Autodesk Inventor part; units mm, degrees
ref_plane "Work Plane1" through (0, 19.05, 0) normal (0, 1, 0) x (-1, 0, 0)
ref_plane "YZ Plane" through (0, 0, 0) normal (1, 0, 0) x (0, 1, 0)
ref_plane "XY Plane" through (0, 0, 0) normal (0, 0, 1) x (1, 0, 0)
sketch "Sketch1" plane through (0, 0, 0) normal (0, 0, 1) x (1, 0, 0)
  line L0 (-106.628, 0) -> (106.628, 0) construction
  line L1 (-63.5, 19.05) -> (63.5, 19.05)
  line L2 (63.5, 19.05) -> (63.5, 15.875)
  line L3 (-63.5, 15.875) -> (-63.5, 19.05)
  line L4 (-63.5, 15.875) -> (-53.34, 15.875)
  line L5 (-53.34, 15.875) -> (-53.34, 16.891)
  line L6 (-53.34, 16.891) -> (-50.8, 16.891)
  line L7 (-50.8, 16.891) -> (-50.8, 15.875)
  line L8 (-50.8, 15.875) -> (0, 15.875)
  line L9 (0, 0) -> (0, 19.05) construction
  line L10 (63.5, 15.875) -> (53.34, 15.875)
  line L11 (53.34, 15.875) -> (53.34, 16.891)
  line L12 (53.34, 16.891) -> (50.8, 16.891)
  line L13 (50.8, 16.891) -> (50.8, 15.875)
  line L14 (50.8, 15.875) -> (0, 15.875)
  dimension "d0" = 127
  dimension "d1" = 38.1
  dimension "d2" = 31.75
  dimension "d3" = 10.16
  dimension "d4" = 2.54
  dimension "d5" = 1.016
revolve "Revolution1" add sketch "Sketch1" angle 360 about axis through (-106.628, 0, 0) along (1, 0, 0)
ref_plane "Work Plane1" through (0, 19.05, 0) normal (0, 1, 0) x (-1, 0, 0)
sketch "Sketch2" plane through (0, 19.05, 0) normal (0, 1, 0) x (-1, 0, 0)
  line L0 (-31.75, 0) -> (9.525, 0) construction
  line L1 (-31.75, -4.7625) -> (9.525, -4.7625)
  line L2 (9.525, 4.7625) -> (-31.75, 4.7625)
  arc A0 (-31.75, 4.7625) -> (-31.75, -4.7625) centre (-31.75, 0) ccw
  arc A1 (9.525, -4.7625) -> (9.525, 4.7625) centre (9.525, 0) ccw
  line L3 (-63.5, 19.05) -> (-63.5, -19.05)
  line L4 (-27.6225, 1.5875) -> (-27.6225, -1.5875)
  line L5 (5.3975, 1.5875) -> (5.3975, -1.5875)
  arc A2 (5.3975, 1.5875) -> (2.2225, 4.7625) centre (2.2225, 1.5875) ccw
  arc A3 (2.2225, -4.7625) -> (5.3975, -1.5875) centre (2.2225, -1.5875) ccw
  arc A4 (-24.4475, 4.7625) -> (-27.6225, 1.5875) centre (-24.4475, 1.5875) ccw
  arc A5 (-27.6225, -1.5875) -> (-24.4475, -4.7625) centre (-24.4475, -1.5875) ccw
  point P0 (0, 0)
  point P1 (-11.1125, 0)
  point P2 (-36.5125, 0)
  point P3 (9.525, 0)
  point P4 (-63.5, 0)
  dimension "d7" = 9.525
  dimension "d8" = 41.275
  dimension "d10" = 33.02
  dimension "d11" = 16.51
  dimension "d12" = 3.175
  dimension "d13" = 3.175
  dimension "d27" = 31.75
extrude "Extrusion1" cut sketch "Sketch2" against normal blind 2.032
extrude "Extrusion2" cut sketch "Sketch2" against normal up to surface contours A5 L4 A4 L2 A2 L5 A3 L1
hole "Hole1" at (-9.525, 19.05, 0) at (31.75, 19.05, 0) direction (0, -1, 0) diameter 2.1565 depth 6.35 tip angle 118
thread "Thread1"
properties part number "InventorNativeNewHilt" material "Aluminum 6061"
CAD build for the part. Positions are in the model's coordinates, mm. A direction names the side the tool comes from. Coordinates: 2 decimals unless noted, no trailing zeros. Loops run counter-clockwise (first coordinate to the right, second up) from the corner with the lowest first, then second, coordinate; pieces in that order, holes last. Notation, with made-up numbers: (-32.5, 22.25) - (-15.5, 22.25) arc R8 cw to (-15.5, 35.25) - close; hole circle Ø5 at (60, 18.5). An arc over 180 degrees is marked (long way). Return JSON: item names as keys, results as strings.
1. Drop flat-ended pins along their axis: pin 1 (1.7 mm diameter, centred on x = 10.5, y = 17, fed in from -Z); pin 2 (6 mm diameter, centred on x = 18.5, y = -9, fed in from +Z); pin 3 (1 mm diameter, centred on x = -17, z = 10, fed in from -Y). Give the stop position or say it passes through.
Result:
{"pin 1": "stops at z = -10.1", "pin 2": "stops at z = 18.08", "pin 3": "stops at y = -16.51"}
2. Band-saw the part on A-A (y = 0). Give the cut face in (x, z) (3 decimals).
Result:
{"outline": "(-63.5, -19.05) - (63.5, -19.05) - (63.5, -15.875) - (53.34, -15.875) - (53.34, -16.891) - (50.8, -16.891) - (50.8, -15.875) - (-50.8, -15.875) - (-50.8, -16.891) - (-53.34, -16.891) - (-53.34, -15.875) - (-63.5, -15.875) - close; (-63.5, 15.875) - (-53.34, 15.875) - (-53.34, 16.891) - (-50.8, 16.891) - (-50.8, 15.875) - (50.8, 15.875) - (50.8, 16.891) - (53.34, 16.891) - (53.34, 15.875) - (63.5, 15.875) - (63.5, 19.05) - (-63.5, 19.05) - close"}
3. 3-axis set-ups, long thin cutter, end or side, ignore diameter. For faces 1 (the cylindrical face through (0.889, 10.241, 16.063)), 2 (the cylindrical face through (-4.4, 16.3, -3.9)), 3 (the cylindrical face through (-52.052, 16.111, 5.074)): which of +Z, -Z, +X, -X, +Y, -Y reach the whole face in a straight line?
Result:
{"face 1": "+X, -X", "face 2": "+Y", "face 3": "none"}
4. Band-saw the part on B-B (z = 14.5). Give the cut face in (x, y).
Result:
{"outline": "(-63.5, -12.36) - (63.5, -12.36) - (63.5, -6.46) - (53.34, -6.46) - (53.34, -8.66) - (50.8, -8.66) - (50.8, -6.46) - (-50.8, -6.46) - (-50.8, -8.66) - (-53.34, -8.66) - (-53.34, -6.46) - (-63.5, -6.46) - close; (-63.5, 6.46) - (-53.34, 6.46) - (-53.34, 8.66) - (-50.8, 8.66) - (-50.8, 6.46) - (50.8, 6.46) - (50.8, 8.66) - (53.34, 8.66) - (53.34, 6.46) - (63.5, 6.46) - (63.5, 12.36) - (-63.5, 12.36) - close"}
5. Probe L1, parallel to X at y = 16, z = 0; L2, parallel to Z at x = -57, y = 0 (3 decimals); L3, parallel to Z at x = 51.4, y = 0. List the from-to ranges inside material, lowest first. Write a range as from..to.
Result:
{"L1": "x = -63.5..-53.34, -50.8..-10.6, -8.45..-5.4, 27.62..30.67, 32.83..50.8, 53.34..63.5", "L2": "z = -19.05..-15.875, 15.875..19.05", "L3": "z = -19.05..-16.89, 16.89..19.05"}
6. Mould opens along X. For faces 4 (the flat face through (63.5, -4, 16)), 5 (the flat face through (11, 17, 4.762)) say: released by +X, released by -X, zero draft, split by the parting line, or undercut.
Result:
{"face 4": "released by +X", "face 5": "undercut"}
